Autodesk Inventor part; units mm, degrees
ref_plane "YZ Plane" through (0, 0, 0) normal (1, 0, 0) x (0, 1, 0)
ref_plane "XZ Plane" through (0, 0, 0) normal (0, 1, 0) x (-1, 0, 0)
ref_plane "XY Plane" through (0, 0, 0) normal (0, 0, 1) x (1, 0, 0)
sketch "Skizze1" plane through (0, 0, 0) normal (0, 0, 1) x (1, 0, 0)
  line L0 (0, 0) -> (56.5, 0) construction
  line L1 (56.5, 0) -> (56.5, -183.5) construction
  line L2 (0, 0) -> (56.5, 0) construction
  line L3 (56.5, 0) -> (56.5, -183.5) construction
  line L4 (56.5, -183.5) -> (0, -183.5) construction
  line L5 (0, -183.5) -> (0, 0) construction
  line L6 (28.25, 0) -> (28.25, 3) construction
  line L7 (28.25, -183.5) -> (28.25, -186.5) construction
  line L8 (28.25, -91.75) -> (1.75, -91.75) construction
  line L9 (28.25, -91.75) -> (-5.75, -91.75) construction
  line L10 (28.25, -91.75) -> (54.75, -91.75) construction
  line L11 (28.25, -91.75) -> (62.25, -91.75) construction
  circle A0 centre (28.25, 3) radius 1.5
  circle A1 centre (28.25, 3) radius 3
  line L12 (28.25, 3) -> (28.25, 10.5) construction
  circle A2 centre (28.25, -186.5) radius 1.5
  circle A3 centre (28.25, -186.5) radius 3
  line L13 (28.25, -186.5) -> (28.25, -194) construction
  circle A4 centre (1.75, -91.75) radius 1.5
  circle A5 centre (1.75, -91.75) radius 3
  circle A6 centre (54.75, -91.75) radius 1.5
  circle A7 centre (54.75, -91.75) radius 3
  line L14 (28.25, -183.5) -> (28.25, -153.093) construction
  line L15 (0, 0) -> (-5.75, -91.75) construction
  line L16 (-5.75, -91.75) -> (0, -183.5) construction
  line L17 (62.25, -91.75) -> (56.25, 0) construction
  arc A8 (0, 0) -> (0, -183.5) centre (729.1304, -91.75) ccw
  line L18 (60.0727, -126.4918) -> (62.25, -91.75) construction
  arc A9 (56.5, 0) -> (0, 0) centre (28.25, -32.753) ccw
  arc A10 (56.5, -183.5) -> (56.5, 0) centre (-672.6304, -91.75) ccw
  arc A11 (0, -183.5) -> (56.5, -183.5) centre (28.25, -150.747) ccw
extrude "Extrusion1" add sketch "Skizze1" along normal blind 3 contours A9 A10 A11 A8
sketch "Skizze2" plane through (0, 0, 0) normal (0, 0, -1) x (-1, 0, 0)
  circle A0 centre (-54.75, -91.75) radius 3 construction
  circle A1 centre (-1.75, -91.75) radius 3 construction
  circle A2 centre (-28.25, -186.5) radius 3 construction
  circle A3 centre (-28.25, 3) radius 3 construction
  arc A4 (0, -183.5) -> (0, 0) centre (-729.1304, -91.75) ccw
  arc A5 (0, 0) -> (-56.5, 0) centre (-28.25, -32.753) ccw
  arc A6 (-56.5, 0) -> (-56.5, -183.5) centre (672.6304, -91.75) ccw
  arc A7 (-56.5, -183.5) -> (0, -183.5) centre (-28.25, -150.747) ccw
  arc A8 (1.8892, -184.5029) -> (1.8892, 1.0029) centre (-729.1304, -91.75) ccw
  arc A9 (-58.3892, -184.5029) -> (1.8892, -184.5029) centre (-28.25, -150.747) ccw
  arc A10 (-58.3892, 1.0029) -> (-58.3892, -184.5029) centre (672.6304, -91.75) ccw
  arc A11 (1.8892, 1.0029) -> (-58.3892, 1.0029) centre (-28.25, -32.753) ccw
  dimension "d25" = 2
extrude "Extrusion2" add sketch "Skizze2" against normal blind 15
sketch "Skizze3" plane through (0, 0, 0) normal (0, 0, -1) x (-1, 0, 0)
  circle A0 centre (-28.25, 3) radius 3
  circle A1 centre (-1.75, -91.75) radius 3
  circle A2 centre (-54.75, -91.75) radius 3
  circle A3 centre (-28.25, -186.5) radius 3
  point P0 (0, 0)
extrude "Extrusion3" add sketch "Skizze3" against normal blind 15
sketch "Skizze4" plane through (28.25, 3, 15) normal (0, 0, 1) x (1, 0, 0)
  circle A0 centre (0, 0) radius 1.5
  circle A1 centre (-26.5, -94.75) radius 3 construction
  circle A2 centre (26.5, -94.75) radius 3 construction
  circle A3 centre (0, -189.5) radius 3 construction
  circle A4 centre (-26.5, -94.75) radius 1.5
  circle A5 centre (26.5, -94.75) radius 1.5
  circle A6 centre (0, -189.5) radius 1.5
  point P0 (-28.25, -3)
  dimension "d30" = 3
  dimension "d31" = 3
  dimension "d32" = 3
  dimension "d33" = 3
extrude "Extrusion4" cut sketch "Skizze4" against normal blind 10
fillet "Rundung1" radius 2 4 edges at (0, 0, 9) (56.5, 0, 9) (56.5, -183.5, 9) (0, -183.5, 9)
fillet "Rundung2" radius 4 8 edges at (64.25, -91.75, 0) (58.3892, 1.0029, 7.5) (28.25, 12.5, 0) (28.25, -196, 0) (-7.75, -91.75, 0) (-1.8892, 1.0029, 7.5) (58.3892, -184.5029, 7.5) (-1.8892, -184.5029, 7.5)
properties part number "armrest"
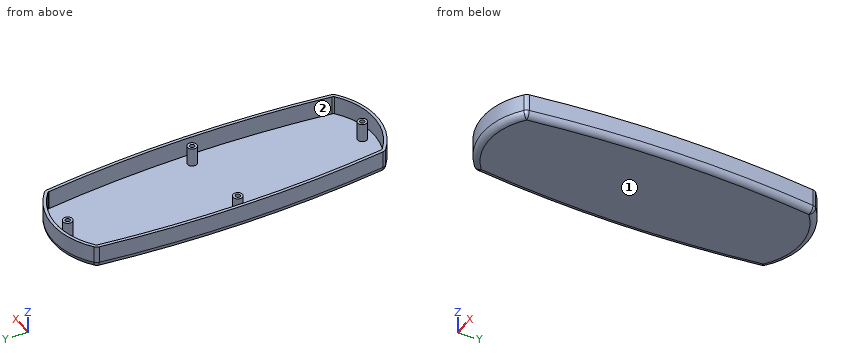
Could you check a few things on this model? Use its own coordinates, in mm. Face numbers are marked on the shaded views. Round coordinates to 2 decimals unless told otherwise and drop trailing zeros. One line per question, with ' | ' between items. Start each with the question number.
(1) Suppose I cut it at A-A on z = 11. Count the separate pieces of the cut face and the enclosed holes in it, then the cut area to 3 significant figures.
(2) For P1, Ø10, axis at x = 36, y = -49, coming from the +Z side; P2, Ø6, axis at x = 37.5, z = 2.5, coming from the -Y side; P3, Ø1.8, axis at x = 1.75, y = -91.75, coming from the +Z side, each with a flat end and sliding along its axis, tell me the tip position at first contact or that it passes through.
(3) Please list where these lines run through material, in increasing order: line 1 along Y through (x, z) = (28.25, 9); line 2 along X through (y, z) = (-98.5, 13.5); line 3 along Y through (x, z) = (54.75, 12.25).
(4) Thinking about a two-plate mould opening in Y: for the marked faces 1 and 2, which applies, +Y half, -Y half, draft (parallel to the pull), parting line (faces both ways), or undercut?
Geometry results:
1) separate pieces: 5 | enclosed holes: 5 | area: 1,080 mm²
2) P1: z = 3 | P2: y = -195.52 | P3: z = 5
3) line 1: -196 to -194, -189.5 to -188, -185 to -183.5, 0 to 1.5, 4.5 to 6, 10.5 to 12.5 | line 2: -7.72 to -5.72, 62.22 to 64.22 | line 3: -187.43 to -184.93, -94.75 to -93.25, -90.25 to -88.75, 1.43 to 3.93
4) face 1: draft | face 2: undercut
